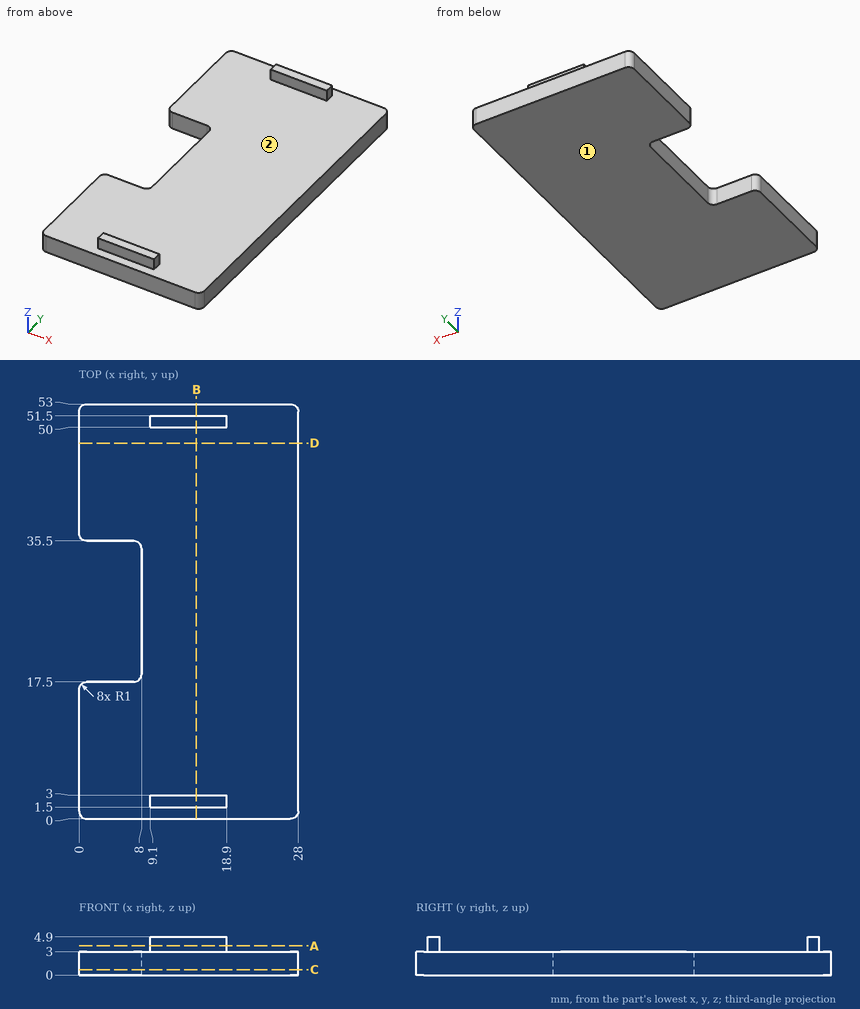
The figure shows three views and two pictorial views of one solid part (mm, origin at its lowest corner). Answer the questions. Give positions to 0.01 mm unless a question says otherwise; leave off trailing zeros. Order: outer loops, then holes, each group sorted by start corner. A loop starts at its lowest first (then second) coordinate and runs counter-clockwise, first axis right, second up. Notation, with made-up numbers: (-24.5, 64.5) -> (18.5, 64.5) arc R23 ccw to (18.5, 84.5) -> close; hole circle Ø8 at (22.5, -25.5). An arc over 180 degrees is marked (long way). Write each question's results on one line, items separated by ' | '.
Q1. Straight lines are drawn through the part: probe 1 along Y at (x, z) = (1.5, 1.3); probe 2 along Y at (x, z) = (18.25, 3.15); probe 3 along Z at (x, y) = (19.5, 41.5). For each, find the intervals that lie inside material, in ascending order. Write a range as from..to.
Checked values:
probe 1: y = 0..17.5, 35.5..53 | probe 2: y = 1.5..3, 50..51.5 | probe 3: z = 0..3
Q2. Each of these flat-tipped pins is pushed along its axis until it touches: P1, Ø1.5, axis at x = 12, y = 15.5, coming from the +Z side; P2, Ø1.2, axis at y = 2, z = 4, coming from the -X side; P3, Ø0.8, axis at y = 2, z = 4.5, coming from the +X side; P4, Ø1, axis at y = 13.5, z = 4, coming from the -X side. Where does it stop, or does it pass through?
Checked values:
P1: stops at z = 3 | P2: stops at x = 9.1 | P3: stops at x = 18.9 | P4: passes through
Q3. Determine the mould class of the marked faces 1 and 2 for opening direction Y: pulls with the +Y half, pulls with the -Y half, needs draft (parallel to the pull), parting line crosses it, or undercut.
Checked values:
face 1: needs draft | face 2: undercut
Q4. The part is cut by section C-C, the plane z = 0.7. Give the vertices of the cut face in (x, y), and give its area (3 significant figures).
Checked values:
outline: (0, 1) arc R1 ccw to (1, 0) -> (27, 0) arc R1 ccw to (28, 1) -> (28, 52) arc R1 ccw to (27, 53) -> (1, 53) arc R1 ccw to (0, 52) -> (0, 36.5) arc R1 ccw to (1, 35.5) -> (7, 35.5) arc R1 cw to (8, 34.5) -> (8, 18.5) arc R1 cw to (7, 17.5) -> (1, 17.5) arc R1 ccw to (0, 16.5) -> close | area: 1,340 mm^2
Q5. The part is cut by section B-B, the plane x = 15. Give the vertices of the cut face in (y, z).
Checked values:
outline: (0, 0) -> (53, 0) -> (53, 3) -> (51.5, 3) -> (51.5, 4.9) -> (50, 4.9) -> (50, 3) -> (3, 3) -> (3, 4.9) -> (1.5, 4.9) -> (1.5, 3) -> (0, 3) -> close
Q6. The part is cut by section D-D, the plane y = 48. Give the vertices of the cut face in (x, z).
Checked values:
outline: (0, 0) -> (28, 0) -> (28, 3) -> (0, 3) -> close
Q7. The part is cut by section A-A, the plane z = 3.75. Give the vertices of the cut face in (x, y).
Checked values:
outline: (9.1, 1.5) -> (18.9, 1.5) -> (18.9, 3) -> (9.1, 3) -> close; (9.1, 50) -> (18.9, 50) -> (18.9, 51.5) -> (9.1, 51.5) -> close
